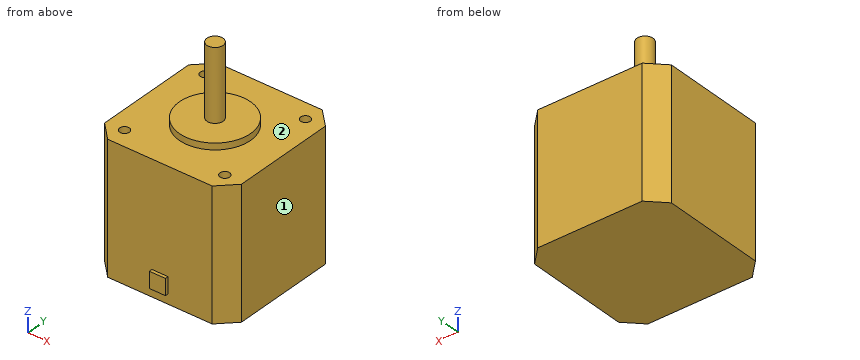
```python
from build123d import *

# Parameters (mm, degrees)
SKETCH1_W           = 42.3
SKETCH1_H           = 42.3
BOSS_EXTRUDE1_DEPTH = 40
SKETCH2_R           = 11
BOSS_EXTRUDE2_DEPTH = 2
SKETCH3_R           = 2.5
BOSS_EXTRUDE3_DEPTH = 22
SKETCH4_R           = 1.5
CUT_EXTRUDE1_DEPTH  = 4.5
CHAMFER1_SIZE       = 5
SKETCH5_W           = 5
SKETCH5_H           = 5
BOSS_EXTRUDE4_DEPTH = 1


with BuildPart() as part:
    # Sketch1 → Boss-Extrude1 (new body)
    with BuildSketch(Plane.XY):
        Rectangle(SKETCH1_W, SKETCH1_H)
    extrude(amount=-BOSS_EXTRUDE1_DEPTH)

    # Sketch2 → Boss-Extrude2 (add)
    with BuildSketch(Plane.XY):
        with Locations(Location((0, 0, 0), (0, 0, 180))):
            Circle(SKETCH2_R)
    extrude(amount=BOSS_EXTRUDE2_DEPTH)

    # Sketch3 → Boss-Extrude3 (add)
    with BuildSketch(Plane.XY.offset(2)):
        Circle(SKETCH3_R)
    extrude(amount=BOSS_EXTRUDE3_DEPTH)

    # Sketch4 → Cut-Extrude1 (cut)
    with BuildSketch(Plane.XY):
        with Locations((-15.5, 15.5)):
            Circle(SKETCH4_R)
        with Locations((15.5, 15.5)):
            Circle(SKETCH4_R)
        with Locations((15.5, -15.5)):
            Circle(SKETCH4_R)
        with Locations((-15.5, -15.5)):
            Circle(SKETCH4_R)
    extrude(amount=-CUT_EXTRUDE1_DEPTH, mode=Mode.SUBTRACT)

    # Chamfer1
    chamfer1_edges = [part.edges().sort_by_distance(p)[0] for p in [
        (-21.15, 21.15, -20),
        (21.15, 21.15, -20),
        (21.15, -21.15, -20),
        (-21.15, -21.15, -20),
    ]]
    chamfer(chamfer1_edges, length=CHAMFER1_SIZE)

    # Sketch5 → Boss-Extrude4 (add)
    with BuildSketch(Plane.XZ.offset(21.15)):
        with Locations((0, -34.5)):
            Rectangle(SKETCH5_W, SKETCH5_H)
    extrude(amount=BOSS_EXTRUDE4_DEPTH)


solid = part.part
```
Build history of the part. All positions in model axes, mm. Face numbers are marked on the shaded views. A direction names the side the tool comes from. Round coordinates to 2 decimals unless told otherwise and drop trailing zeros. Order: outer loops, then holes, each group sorted by start corner. A loop starts at its lowest first (then second) coordinate and runs counter-clockwise, first axis right, second up. Notation, with made-up numbers: (80.5, 83.25) - (107.5, 83.25) arc R30 ccw to (107.5, 115.25) - close; hole circle Ø5 at (32, 33.25). An arc over 180 degrees is marked (long way). Use a Markdown table: item, result.
1) Tool access for the marked faces 1 and 2: list every direction of +Z, -Z, +X, -X, +Y, -Y with a clear straight run to the whole face (end or side of a thin tool).
Recorded:
| item | result |
|---|---|
| face 1 | +Z, -Z, +X, +Y, -Y |
| face 2 | +Z |
2) Saw through at B-B on z = -36. Write the cut outline in (x, y), and give its area (3 significant figures).
Recorded:
| item | result |
|---|---|
| outline | (-21.15, -16.15) - (-16.15, -21.15) - (-2.5, -21.15) - (-2.5, -22.15) - (2.5, -22.15) - (2.5, -21.15) - (16.15, -21.15) - (21.15, -16.15) - (21.15, 16.15) - (16.15, 21.15) - (-16.15, 21.15) - (-21.15, 16.15) - close |
| area | 1,740 mm² |
3) Saw through at A-A on x = 0. Write the cut outline in (y, z).
Recorded:
| item | result |
|---|---|
| outline | (-22.15, -37) - (-21.15, -37) - (-21.15, -40) - (21.15, -40) - (21.15, 0) - (11, 0) - (11, 2) - (2.5, 2) - (2.5, 24) - (-2.5, 24) - (-2.5, 2) - (-11, 2) - (-11, 0) - (-21.15, 0) - (-21.15, -32) - (-22.15, -32) - close |
4) Saw through at D-D on z = -22. Write the cut outline in (x, y).
Recorded:
| item | result |
|---|---|
| outline | (-21.15, -16.15) - (-16.15, -21.15) - (16.15, -21.15) - (21.15, -16.15) - (21.15, 16.15) - (16.15, 21.15) - (-16.15, 21.15) - (-21.15, 16.15) - close |
5) Wall check: L1, parallel to Y at x = 15.5, z = -2; L2, parallel to Y at x = -15, z = -2; L3, parallel to Y at x = -5.5, z = -22.5. Give the ranges that are in metal, low to high.
Recorded:
| item | result |
|---|---|
| L1 | y = -21.15 to -17, -14 to 14, 17 to 21.15 |
| L2 | y = -21.15 to -16.91, -14.09 to 14.09, 16.91 to 21.15 |
| L3 | y = -21.15 to 21.15 |
6) Flat gauge pins, fed straight in: pin 1 Ø0.9 at (x, y) = (16, 15.5) entering from +Z; pin 2 Ø0.8 at (y, z) = (-21.5, -34.5) entering from +X; pin 3 Ø5 at (x, y) = (-15.5, -15.5) entering from +Z. Where does each tip first touch, or does it go through?
Recorded:
| item | result |
|---|---|
| pin 1 | stops at z = -4.5 |
| pin 2 | stops at x = 16.2 |
| pin 3 | stops at z = 0 |
7) Saw through at C-C on y = 0. Write the cut outline in (x, z).
Recorded:
| item | result |
|---|---|
| outline | (-21.15, -40) - (21.15, -40) - (21.15, 0) - (11, 0) - (11, 2) - (2.5, 2) - (2.5, 24) - (-2.5, 24) - (-2.5, 2) - (-11, 2) - (-11, 0) - (-21.15, 0) - close |
